from build123d import *

# Parameters (mm, degrees)
SKETCH1_W           = 103
SKETCH1_H           = 103
BOSS_EXTRUDE1_DEPTH = 15
SKETCH3_W           = 15
SKETCH3_H           = 103
BOSS_EXTRUDE2_DEPTH = 5
CUT_EXTRUDE1_DEPTH  = 5
SKETCH5_W           = 86
SKETCH5_H           = 75
CUT_EXTRUDE2_DEPTH  = 157.949036314
CUT_EXTRUDE5_REACH  = 170.888
SKETCH9_W           = 10
SKETCH9_H           = 10


with BuildPart() as part:
    # Sketch1 → Boss-Extrude1 (new body)
    with BuildSketch(Plane.XY):
        with Locations((51.5, -51.5)):
            Rectangle(SKETCH1_W, SKETCH1_H)
    extrude(amount=BOSS_EXTRUDE1_DEPTH)

    # Sketch3 → Boss-Extrude2 (add)
    with BuildSketch(Plane(origin=(0, 0, 0), x_dir=(-1, 0, 0), z_dir=(0, 0, -1))):
        with Locations((7.5, -51.5)):
            Rectangle(SKETCH3_W, SKETCH3_H)
        with Locations((-110.5, -51.5)):
            Rectangle(SKETCH3_W, SKETCH3_H)
    extrude(amount=-BOSS_EXTRUDE2_DEPTH)

    # Sketch4 → Cut-Extrude1 (cut)
    with BuildSketch(Plane(origin=(0, 0, 0), x_dir=(-1, 0, 0), z_dir=(0, 0, -1))):
        Polygon((-51.5, -51.5), (-101.5, -1.5), (-101.5, -101.5), align=None)
        Polygon((-1.5, -1.5), (-101.5, -1.5), (-51.5, -51.5), align=None)
        Polygon((-1.5, -1.5), (-51.5, -51.5), (-1.5, -101.5), align=None)
        Polygon((-1.5, -101.5), (-51.5, -51.5), (-101.5, -101.5), align=None)
    extrude(amount=-CUT_EXTRUDE1_DEPTH, mode=Mode.SUBTRACT)

    # Sketch5 → Cut-Extrude2 (cut, through all)
    with BuildSketch(Plane(origin=(0, 0, 5), x_dir=(-1, 0, 0), z_dir=(0, 0, -1))):
        with Locations((-51.5, -51.5)):
            Rectangle(SKETCH5_W, SKETCH5_H)
    extrude(amount=-CUT_EXTRUDE2_DEPTH, mode=Mode.SUBTRACT)

    # Cut-Extrude5: up to this face of the body (flat: up to its plane)
    cut_extrude5_end = Plane(part.part.faces().sort_by_distance((8.5, -51.5, 10))[0])
    # Sketch9 → Cut-Extrude5 (cut, up to the picked face)
    with BuildSketch(Plane.ZY.offset(15), mode=Mode.PRIVATE) as cut_extrude5_sk1:
        with Locations((0, -51.5)):
            Rectangle(SKETCH9_W, SKETCH9_H)
    cut_extrude5_tool1 = split(extrude(cut_extrude5_sk1.sketch, amount=-CUT_EXTRUDE5_REACH, mode=Mode.PRIVATE), bisect_by=cut_extrude5_end, keep=Keep.BOTH, mode=Mode.PRIVATE)
    cut_extrude5 = cut_extrude5_tool1.solids().sort_by(Axis((-15, -51.5, 0), (1, 0, 0)))[0]
    add(cut_extrude5, mode=Mode.SUBTRACT)

    # Mirror1: Cut-Extrude5 across plane
    add(cut_extrude5.mirror(Plane.ZY.offset(-51.5)), mode=Mode.SUBTRACT)


solid = part.part
Geometry check sheet. Reference: the model listing, model coordinates, mm. A direction names the side the tool comes from. Give positions to 0.01 mm unless a question says otherwise; leave off trailing zeros. Write each loop counter-clockwise with the first axis right and the second up, starting at its lowest first coordinate (ties: lowest second). Pieces come first, ordered by that corner, then holes. Notation, with made-up numbers: M 64,35.25 L 108,35.25 A17 cw 108,43.25 Z; hole C 71,75.25 d5. An arc over 180 degrees is marked long. One line per question, with ' | ' between items.
1. Gauge pin test, flat ends, axial feed: pin 1 (16.5 mm diameter, centred on x = -8.5, y = -71, fed in from +Z); pin 2 (2 mm diameter, centred on y = -29.5, z = 10, fed in from -X); pin 3 (4 mm diameter, centred on x = -5.5, z = 1.5, fed in from +Y); pin 4 (5 mm diameter, centred on y = -76.5, z = 11.5, fed in from +X). Record the tip position at first contact, or that the pin passes through.
Ans:
pin 1: z = 5 | pin 2: x = 0 | pin 3: y = 0 | pin 4: x = 103
2. Cross-section at A-A (x = 108). Enter the section's corners in (y, z).
Ans:
outline: M -103,0 L -56.5,0 L -56.5,5 L -103,5 Z; M -46.5,0 L 0,0 L 0,5 L -46.5,5 Z
3. Mould release check, pull along X, two halves, no side actions. Record for faces 5 (the face through (47, -1, 0)), 6 (the face through (52, -101.5, 2)), 7 (the face through (103, -52, 10)): released by +X, released by -X, zero draft, split by the parting line, or undercut.
Ans:
face 5: zero draft | face 6: undercut | face 7: released by +X
4. Cross-section at D-D (x = 6). Enter the section's corners in (y, z).
Ans:
outline: M -103,0 L -101.5,0 L -101.5,5 L -1.5,5 L -1.5,0 L 0,0 L 0,15 L -103,15 Z
5. Cross-section at C-C (z = 11.75). Enter the section's corners in (x, y), plus the area to 3 significant figures.
Ans:
outline: M 0,-103 L 103,-103 L 103,0 L 0,0 Z; hole M 8.5,-89 L 94.5,-89 L 94.5,-14 L 8.5,-14 Z | area: 4,160 mm2
6. Scan lines: line 1 along X through (y, z) = (-68.5, 7.75); line 2 along X through (y, z) = (-45, 1.5); line 3 along Y through (x, z) = (42, 4.25). Record each from-to range of solid material in increasing order. Write a range as from..to.
Ans:
line 1: 0..8.5, 94.5..103 | line 2: -15..1.5, 101.5..118 | line 3: -103..-101.5, -1.5..0
7. Set-up check for faces 1 (the face through (-7, -79, 5)), 2 (the face through (1.5, -24, 2)), 3 (the face through (52, 0, 7)), 4 (the face through (52, -89, 10)): record each of +Z, -Z, +X, -X, +Y, -Y from which the full face is reachable in a straight line by a thin tool's end or side.
Ans:
face 1: +Z, -X, +Y, -Y | face 2: -Z | face 3: +Z, -Z, +X, -X, +Y | face 4: +Z, -Z
8. Cross-section at B-B (y = -59.5). Enter the section's corners in (x, z).
Ans:
outline: M -15,0 L 1.5,0 L 1.5,5 L 8.5,5 L 8.5,15 L 0,15 L 0,5 L -15,5 Z; M 94.5,5 L 101.5,5 L 101.5,0 L 118,0 L 118,5 L 103,5 L 103,15 L 94.5,15 Z
